```python
from build123d import *

# Parameters (mm, degrees)
SKETCH1_W           = 20
SKETCH1_H           = 15
BOSS_EXTRUDE1_DEPTH = 3
SKETCH2_W           = 10
SKETCH2_H           = 4
BOSS_EXTRUDE2_DEPTH = 13
SKETCH4_W           = 10
SKETCH4_H           = 4
CUT_EXTRUDE3_DEPTH  = 4
SKETCH3_R           = 2
CUT_EXTRUDE4_DEPTH  = 13


with BuildPart() as part:
    # Sketch1 → Boss-Extrude1 (new body)
    with BuildSketch(Plane.XY):
        with Locations((-10, 7.5)):
            Rectangle(SKETCH1_W, SKETCH1_H)
    extrude(amount=BOSS_EXTRUDE1_DEPTH)

    # Sketch2 → Boss-Extrude2 (add)
    with BuildSketch(Plane.XY.offset(3)):
        with Locations((-10, 10)):
            Rectangle(SKETCH2_W, SKETCH2_H)
    extrude(amount=BOSS_EXTRUDE2_DEPTH)

    # Sketch4 → Cut-Extrude3 (cut, through all)
    with BuildSketch(Plane.XY.offset(3)):
        with Locations((-10, 5)):
            Rectangle(SKETCH4_W, SKETCH4_H)
    extrude(amount=-CUT_EXTRUDE3_DEPTH, mode=Mode.SUBTRACT)

    # Sketch3 → Cut-Extrude4 (cut, through all)
    with BuildSketch(Plane(origin=(0, 12, 0), x_dir=(1, 0, 0), z_dir=(0, 1, 0))):
        with Locations((-10, -11)):
            Circle(SKETCH3_R)
    extrude(amount=-CUT_EXTRUDE4_DEPTH, mode=Mode.SUBTRACT)


solid = part.part
```
Input: part model. Units: mm. Frame: model coordinates. A direction names the side the tool comes from. Give positions to 0.01 mm unless a question says otherwise; leave off trailing zeros. Loops run counter-clockwise (first coordinate to the right, second up) from the corner with the lowest first, then second, coordinate; pieces in that order, holes last. Notation, with made-up numbers: (52, 8) -> (72, 8) arc R18 cw to (72, 13) -> close; hole circle Ø4 at (-5.75, 45). An arc over 180 degrees is marked (long way). Use a Markdown table: item, result.
Q1. First-contact query: P1, Ø3, axis at y = 6.5, z = 3.5, coming from the -X side; P2, Ø4, axis at y = 10.5, z = 13, coming from the -X side; P3, Ø3, axis at y = 6, z = 9, coming from the +X side; P4, Ø3, axis at y = 9.5, z = 10, coming from the +X side. Flat tips, straight axial feed; report the tip coordinate or a pass-through.
Entries:
| item | result |
|---|---|
| P1 | stops at x = -20 |
| P2 | stops at x = -15 |
| P3 | passes through |
| P4 | stops at x = -5 |
Q2. Section query B-B, the plane x = -10. Return the cut outline in (y, z).
Entries:
| item | result |
|---|---|
| outline | (0, 0) -> (3, 0) -> (3, 3) -> (0, 3) -> close; (7, 0) -> (15, 0) -> (15, 3) -> (12, 3) -> (12, 9) -> (8, 9) -> (8, 3) -> (7, 3) -> close; (8, 13) -> (12, 13) -> (12, 16) -> (8, 16) -> close |
Q3. Ray query, probe 1 along Z at (x, y) = (-10, 10.1); probe 2 along X at (y, z) = (9.55, 11); probe 3 along X at (y, z) = (8.25, 5.25). Return the intervals inside material, ascending. Write a range as from..to.
Entries:
| item | result |
|---|---|
| probe 1 | z = 0..9, 13..16 |
| probe 2 | x = -15..-12, -8..-5 |
| probe 3 | x = -15..-5 |
Q4. Section query D-D, the plane y = 10. Return the cut outline in (x, z).
Entries:
| item | result |
|---|---|
| outline | (-20, 0) -> (0, 0) -> (0, 3) -> (-5, 3) -> (-5, 16) -> (-15, 16) -> (-15, 3) -> (-20, 3) -> close; hole circle Ø4 at (-10, 11) |
Q5. Section query A-A, the plane y = 3.5. Return the cut outline in (x, z).
Entries:
| item | result |
|---|---|
| outline | (-20, 0) -> (-15, 0) -> (-15, 3) -> (-20, 3) -> close; (-5, 0) -> (0, 0) -> (0, 3) -> (-5, 3) -> close |
Q6. Access query for faces 4 (the flat face through (-5, 5, 2)), 5 (the flat face through (-15, 10, 9)), 6 (the flat face through (-5, 10, 9)). Directions: +Z, -Z, +X, -X, +Y, -Y. A direction counts if a zero-diameter tool reaches every point of the face in a straight line with its end or side. Return the directions, or none.
Entries:
| item | result |
|---|---|
| face 4 | +Z, -Z |
| face 5 | +Z, -X, +Y, -Y |
| face 6 | +Z, +X, +Y, -Y |
Q7. Section query C-C, the plane z = 11. Return the cut outline in (x, y).
Entries:
| item | result |
|---|---|
| outline | (-15, 8) -> (-12, 8) -> (-12, 12) -> (-15, 12) -> close; (-8, 8) -> (-5, 8) -> (-5, 12) -> (-8, 12) -> close |
Q8. Pull-direction query (Y, two-part tool) for faces 1 (the flat face through (-10, 8, 0)), 2 (the flat face through (-10, 8, 8)), 3 (the flat face through (-10, 3, 2)); classes: pulls with the +Y half, pulls with the -Y half, needs draft (parallel to the pull), parting line crosses it, or undercut.
Entries:
| item | result |
|---|---|
| face 1 | needs draft |
| face 2 | pulls with the -Y half |
| face 3 | undercut |
